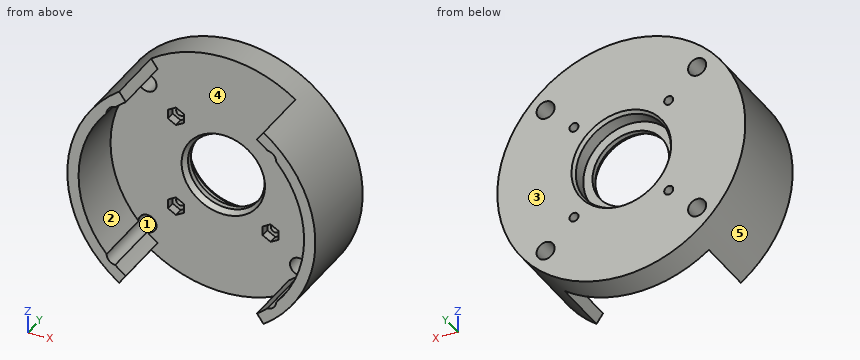
from build123d import *

# Parameters (mm, degrees)
SKETCH_1_R          = 55
EXTRUDE_1_DEPTH     = 40
SKETCH_2_R          = 50
CUT_EXTRUDE_1_DEPTH = 27
SKETCH_3_R          = 17
CUT_EXTRUDE_2_DEPTH = 14
SKETCH_4_R          = 4
CUT_EXTRUDE_3_DEPTH = 41
SKETCH1_R           = 21.1
CUT_EXTRUDE1_DEPTH  = 8
CHAMFER1_SIZE       = 1
CHAMFER1_SIZE2      = 1.732050808
SKETCH2_R           = 2
CUT_EXTRUDE2_DEPTH  = 41
CUT_EXTRUDE3_DEPTH  = 4
CUT_EXTRUDE4_DEPTH  = 27
CHAMFER2_SIZE       = 1.5
CHAMFER2_SIZE2      = 2.598076211


with BuildPart() as part:
    # Эскиз1 → Бобышка-Вытянуть1 (new body)
    with BuildSketch(Plane(origin=(0, 0, 0), x_dir=(1, 0, 0), z_dir=(0, 1, 0))):
        with Locations(Location((0, 0, 0), (0, 0, 270))):  # turned: the seam where the file's is
            Circle(SKETCH_1_R)
    extrude(amount=EXTRUDE_1_DEPTH)

    # Эскиз2 → Вырез-Вытянуть1 (cut)
    with BuildSketch(Plane.XZ):
        with Locations(Location((0, 0, 0), (0, 0, 270))):  # turned: the seam where the file's is
            Circle(SKETCH_2_R)
    extrude(amount=-CUT_EXTRUDE_1_DEPTH, mode=Mode.SUBTRACT)

    # Эскиз3 → Вырез-Вытянуть2 (cut, through all)
    with BuildSketch(Plane.XZ.offset(-27)):
        with Locations(Location((0, 0, 0), (0, 0, 270))):  # turned: the seam where the file's is
            Circle(SKETCH_3_R)
    extrude(amount=-CUT_EXTRUDE_2_DEPTH, mode=Mode.SUBTRACT)

    # Эскиз4 → Вырез-Вытянуть3 (cut, through all)
    with BuildSketch(Plane(origin=(0, 40, 0), x_dir=(1, 0, 0), z_dir=(0, 1, 0))):
        with Locations(Location((33.591727056, -32.872418125, 0), (0, 0, 270))):  # turned: the seam where the file's is
            Circle(SKETCH_4_R)
        with Locations(Location((-33.591727056, -32.872418125, 0), (0, 0, 270))):  # turned: the seam where the file's is
            Circle(SKETCH_4_R)
        with Locations(Location((-33.591727056, 32.872418125, 0), (0, 0, 270))):  # turned: the seam where the file's is
            Circle(SKETCH_4_R)
        with Locations(Location((33.591727056, 32.872418125, 0), (0, 0, 270))):  # turned: the seam where the file's is
            Circle(SKETCH_4_R)
    extrude(amount=-CUT_EXTRUDE_3_DEPTH, mode=Mode.SUBTRACT)

    # Sketch1 → Cut-Extrude1 (cut)
    with BuildSketch(Plane(origin=(0, 40, 0), x_dir=(1, 0, 0), z_dir=(0, 1, 0))):
        with Locations(Location((0, 0, 0), (0, 0, 270))):  # turned: the seam where the file's is
            Circle(SKETCH1_R)
    extrude(amount=-CUT_EXTRUDE1_DEPTH, mode=Mode.SUBTRACT)

    # Chamfer1
    chamfer1_edges = [part.edges().sort_by_distance(p)[0] for p in [
        (0, 40, -21.1),
    ]]
    chamfer1_side = [part.faces().sort_by_distance(p)[0] for p in [
        (0, 40, -53.444365081),
    ]]
    chamfer(chamfer1_edges, length=CHAMFER1_SIZE, length2=CHAMFER1_SIZE2, reference=chamfer1_side[0])

    # Sketch2 → Cut-Extrude2 (cut, through all)
    with BuildSketch(Plane(origin=(0, 40, 0), x_dir=(1, 0, 0), z_dir=(0, 1, 0))):
        with Locations(Location((21, 21, 0), (0, 0, 270))):  # turned: the seam where the file's is
            Circle(SKETCH2_R)
        with Locations(Location((-21, 21, 0), (0, 0, 270))):  # turned: the seam where the file's is
            Circle(SKETCH2_R)
        with Locations(Location((21, -21, 0), (0, 0, 270))):  # turned: the seam where the file's is
            Circle(SKETCH2_R)
        with Locations(Location((-21, -21, 0), (0, 0, 270))):  # turned: the seam where the file's is
            Circle(SKETCH2_R)
    extrude(amount=-CUT_EXTRUDE2_DEPTH, mode=Mode.SUBTRACT)

    # Sketch3 → Cut-Extrude3 (cut)
    with BuildSketch(Plane.XZ.offset(-27)):
        Polygon((-21, -16.9), (-24.550704156, -18.95), (-24.550704156, -23.05), (-21, -25.1), (-17.449295844, -23.05), (-17.449295844, -18.95), align=None)
        Polygon((-21, 25.1), (-24.550704156, 23.05), (-24.550704156, 18.95), (-21, 16.9), (-17.449295844, 18.95), (-17.449295844, 23.05), align=None)
        Polygon((24.550704156, 23.05), (21, 25.1), (17.449295844, 23.05), (17.449295844, 18.95), (21, 16.9), (24.550704156, 18.95), align=None)
        Polygon((24.550704156, -18.95), (21, -16.9), (17.449295844, -18.95), (17.449295844, -23.05), (21, -25.1), (24.550704156, -23.05), align=None)
    extrude(amount=-CUT_EXTRUDE3_DEPTH, mode=Mode.SUBTRACT)

    # Sketch4 → Cut-Extrude4 (cut)
    with BuildSketch(Plane.XZ):
        with BuildLine():
            Line((32, -44.732538493), (29.090909091, -40.665944084))
            ThreePointArc((29.090909091, -40.665944084), (0, -50), (-29.090909091, -40.665944084))
            Line((-29.090909091, -40.665944084), (-32, -44.732538493))
            ThreePointArc((-32, -44.732538493), (0, -55), (32, -44.732538493))
        make_face()
        with BuildLine():
            Line((32, 44.732538493), (29.090909091, 40.665944084))
            ThreePointArc((29.090909091, 40.665944084), (0, 50), (-29.090909091, 40.665944084))
            Line((-29.090909091, 40.665944084), (-32, 44.732538493))
            ThreePointArc((-32, 44.732538493), (0, 55), (32, 44.732538493))
        make_face()
    extrude(amount=-CUT_EXTRUDE4_DEPTH, mode=Mode.SUBTRACT)

    # Chamfer2
    chamfer2_edges = [part.edges().sort_by_distance(p)[0] for p in [
        (0, 27, 17),
    ]]
    chamfer2_side = [part.faces().sort_by_distance(p)[0] for p in [
        (29.336369105, 27, 43.564176197),
    ]]
    chamfer(chamfer2_edges, length=CHAMFER2_SIZE, length2=CHAMFER2_SIZE2, reference=chamfer2_side[0])


solid = part.part
Design review of the part built by this model. Coordinates are the model's own, in mm. Face numbers are marked on the shaded views. A direction names the side the tool comes from. Give positions to 0.01 mm unless a question says otherwise; leave off trailing zeros. Order: outer loops, then holes, each group sorted by start corner. A loop starts at its lowest first (then second) coordinate and runs counter-clockwise, first axis right, second up.
1. Add section D-D, the plane z = 26.5. State the section outline as (x, y) points, then the cut area to 3 significant figures.
Solution:
outline: (-48.19, 0) - (-42.4, 0) - (-42.4, 27) - (42.4, 27) - (42.4, 0) - (48.19, 0) - (48.19, 40) - (-48.19, 40) - close
area: 1,570 mm2
2. Add section A-A, the plane z = 0. State the section outline as (x, y) points, then the cut area to 3 significant figures.
Solution:
outline: (-55, 0) - (-50, 0) - (-50, 27) - (-18.5, 27) - (-17, 29.6) - (-17, 32) - (-21.1, 32) - (-21.1, 38.27) - (-22.1, 40) - (-55, 40) - close; (17, 29.6) - (18.5, 27) - (50, 27) - (50, 0) - (55, 0) - (55, 40) - (22.1, 40) - (21.1, 38.27) - (21.1, 32) - (17, 32) - close
area: 1,190 mm2
3. For pin 1 Ø2 at (y, z) = (28.5, -22) entering from +X; pin 2 Ø4.5 at (y, z) = (28.5, -21) entering from -X; pin 3 Ø6.5 at (x, z) = (21, 21) entering from -Y; pin 4 Ø6.5 at (x, z) = (-33.59, -32.87) entering from +Y, all flat-tipped, find the tip position at first contact; note any pin that passes through.
Solution:
pin 1: stops at x = 50.83
pin 2: stops at x = -51.71
pin 3: stops at y = 31
pin 4: passes through
4. Mouldability with a two-part tool opening along Z and no side actions: class the marked faces 3, 4 and 5 as +Z half, -Z half, draft (parallel to the pull), parting line (faces both ways), or undercut.
Solution:
face 3: draft
face 4: undercut
face 5: parting line
5. To check wall thickness, follow L1, parallel to Y at x = 23.5, z = -0.5; L2, parallel to X at y = 15, z = 21.5; L3, parallel to Z at x = 8, y = 33. State the ranges of each line that lie inside material, in increasing order.
Solution:
L1: y = 27 to 40
L2: x = -50.62 to -45.14, 45.14 to 50.62
L3: z = -54.42 to -19.52, 19.52 to 54.42
6. Add section B-B, the plane y = 18.5. State the section outline as (x, z) points, then the cut area to 3 significant figures.
Solution:
outline: (-37.59, -32.97) arc R50 cw to (-37.59, 32.97) arc R4 cw to (-33.77, 36.87) arc R50 cw to (-29.09, 40.67) - (-32, 44.73) arc R55 ccw to (-32, -44.73) - (-29.09, -40.67) arc R50 cw to (-33.77, -36.87) arc R4 cw to start; (29.09, -40.67) - (32, -44.73) arc R55 ccw to (32, 44.73) - (29.09, 40.67) arc R50 cw to (33.77, 36.87) arc R4 cw to (37.59, 32.97) arc R50 cw to (37.59, -32.97) arc R4 cw to (33.77, -36.87) arc R50 cw to start
area: 982 mm2
7. Tool access review of the marked faces 1 and 2: name each direction out of +Z, -Z, +X, -X, +Y, -Y from which nothing blocks a thin tool from reaching the whole face with its end or side.
Solution:
face 1: +Y, -Y
face 2: -Y
8. Add section C-C, the plane y = 36. State how many separate pieces and enclosed holes the cut face has, then the cut area to 3 significant figures.
Solution:
separate pieces: 1
enclosed holes: 9
area: 7,850 mm2
